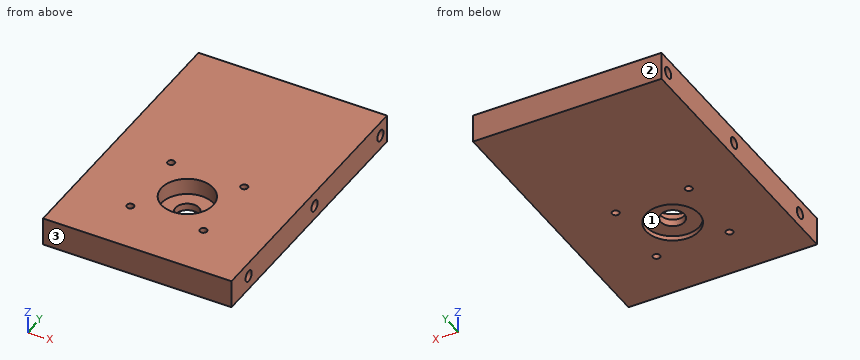
from build123d import *

# Parameters (mm, degrees)
CROQUIS1_W              = 80
CROQUIS1_H              = 110
CROQUIS1_R              = 5
CROQUIS1_R_2            = 1.5
SALIENTE_EXTRUIR1_DEPTH = 12
CROQUIS4_R              = 11.25
CORTAR_EXTRUIR2_DEPTH   = 2
CROQUIS5_R              = 2.35
CORTAR_EXTRUIR3_DEPTH   = 5
CORTAR_EXTRUIR4_START   = -5
CROQUIS6_R              = 2.35
CORTAR_EXTRUIR4_DEPTH   = 5
CROQUIS7_R              = 11
CORTAR_EXTRUIR5_DEPTH   = 7
CROQUIS8_W              = 80
CROQUIS8_H              = 8
SALIENTE_EXTRUIR2_DEPTH = 12


with BuildPart() as part:
    # Croquis1 → Saliente-Extruir1 (new body)
    with BuildSketch(Plane.XY):
        with Locations((40, 55)):
            Rectangle(CROQUIS1_W, CROQUIS1_H)
        with Locations((40, 30)):
            Circle(CROQUIS1_R, mode=Mode.SUBTRACT)
        with Locations((55.5, 45.5)):
            Circle(CROQUIS1_R_2, mode=Mode.SUBTRACT)
        with Locations((24.5, 45.5)):
            Circle(CROQUIS1_R_2, mode=Mode.SUBTRACT)
        with Locations((24.5, 14.5)):
            Circle(CROQUIS1_R_2, mode=Mode.SUBTRACT)
        with Locations((55.5, 14.5)):
            Circle(CROQUIS1_R_2, mode=Mode.SUBTRACT)
    extrude(amount=SALIENTE_EXTRUIR1_DEPTH)

    # Croquis4 → Cortar-Extruir2 (cut)
    with BuildSketch(Plane(origin=(0, 0, 0), x_dir=(-1, 0, 0), z_dir=(0, 0, -1))):
        with Locations((-40, 30)):
            Circle(CROQUIS4_R)
    extrude(amount=-CORTAR_EXTRUIR2_DEPTH, mode=Mode.SUBTRACT)

    # Croquis5 → Cortar-Extruir3 (cut)
    with BuildSketch(Plane(origin=(80, 0, 0), x_dir=(0, 0, -1), z_dir=(1, 0, 0))):
        with Locations(Location((-6, 105, 0), (0, 0, 90))):
            Circle(CROQUIS5_R)
        with Locations(Location((-6, 55, 0), (0, 0, 90))):
            Circle(CROQUIS5_R)
        with Locations(Location((-6, 5, 0), (0, 0, 90))):
            Circle(CROQUIS5_R)
    extrude(amount=-CORTAR_EXTRUIR3_DEPTH, mode=Mode.SUBTRACT)

    # Croquis6 → Cortar-Extruir4 (cut)
    with BuildSketch(Plane.ZY.offset(CORTAR_EXTRUIR4_START)):
        with Locations(Location((6, 105, 0), (0, 0, 90))):
            Circle(CROQUIS6_R)
        with Locations(Location((6, 55, 0), (0, 0, 90))):
            Circle(CROQUIS6_R)
        with Locations(Location((6, 5, 0), (0, 0, 90))):
            Circle(CROQUIS6_R)
    extrude(amount=CORTAR_EXTRUIR4_DEPTH, mode=Mode.SUBTRACT)

    # Croquis7 → Cortar-Extruir5 (cut)
    with BuildSketch(Plane.XY.offset(12)):
        with Locations((40, 30)):
            Circle(CROQUIS7_R)
    extrude(amount=-CORTAR_EXTRUIR5_DEPTH, mode=Mode.SUBTRACT)

    # Croquis8 → Saliente-Extruir2 (add)
    with BuildSketch(Plane.XY.offset(12)):
        with Locations((40, -4)):
            Rectangle(CROQUIS8_W, CROQUIS8_H)
    extrude(amount=-SALIENTE_EXTRUIR2_DEPTH)


solid = part.part
Design review of the part built by this model. Coordinates are the model's own, in mm. Face numbers are marked on the shaded views. Round coordinates to 2 decimals unless told otherwise and drop trailing zeros. Write each loop counter-clockwise with the first axis right and the second up, starting at its lowest first coordinate (ties: lowest second). Pieces come first, ordered by that corner, then holes. Notation, with made-up numbers: (36, 63.25) - (87, 63.25) arc R8 cw to (87, 71.25) - close; hole circle Ø6 at (56.5, -24). An arc over 180 degrees is marked (long way). Return JSON: item names as keys, results as strings. Group by question number.
Item 1: We need section B-B on y = 55. Write out the cut boundary in (x, z).
Item 2: We need section A-A on y = 14.5. Write out the cut boundary in (x, z).
Item 3: The part is to be moulded in two halves that separate along Y. For the marked faces 1, 2 and 3, say which applies: pulls with the +Y half, pulls with the -Y half, needs draft (parallel to the pull), parting line crosses it, or undercut.
Item 4: Insertion check: P1, Ø1.4, axis at y = 5.5, z = 6.5, coming from the -X side; P2, Ø3, axis at y = 5, z = 6, coming from the +X side; P3, Ø1.8, axis at x = 24.5, y = 45.5, coming from the -Z side; P4, Ø11, axis at x = 44, y = 31.5, coming from the -Z side. Each pin has a flat end and moves straight along its axis. Give the tip position at first contact, or say it passes through.
Item 5: For probe 1 along X at (y, z) = (15, 9.5); probe 2 along Z at (x, y) = (2, 55); probe 3 along Y at (x, z) = (54.5, 5.75), list the stretches that pass through material, from the lowest coordinate up. Write a range as [from, to].
Model answer:
{
 "1": {"outline": "(0, 0) - (80, 0) - (80, 3.65) - (75, 3.65) - (75, 8.35) - (80, 8.35) - (80, 12) - (0, 12) - (0, 8.35) - (5, 8.35) - (5, 3.65) - (0, 3.65) - close"},
 "2": {"outline": "(0, 0) - (23, 0) - (23, 12) - (0, 12) - close; (26, 0) - (54, 0) - (54, 12) - (26, 12) - close; (57, 0) - (80, 0) - (80, 12) - (57, 12) - close"},
 "3": {"face 1": "undercut", "face 2": "pulls with the +Y half", "face 3": "pulls with the -Y half"},
 "4": {"P1": "stops at x = 5", "P2": "stops at x = 75", "P3": "passes through", "P4": "stops at z = 2"},
 "5": {"probe 1": "x = [0, 23.09], [25.91, 54.09], [56.91, 80]", "probe 2": "z = [0, 3.65], [8.35, 12]", "probe 3": "y = [-8, 13.38], [15.62, 44.38], [46.62, 110]"}
}
